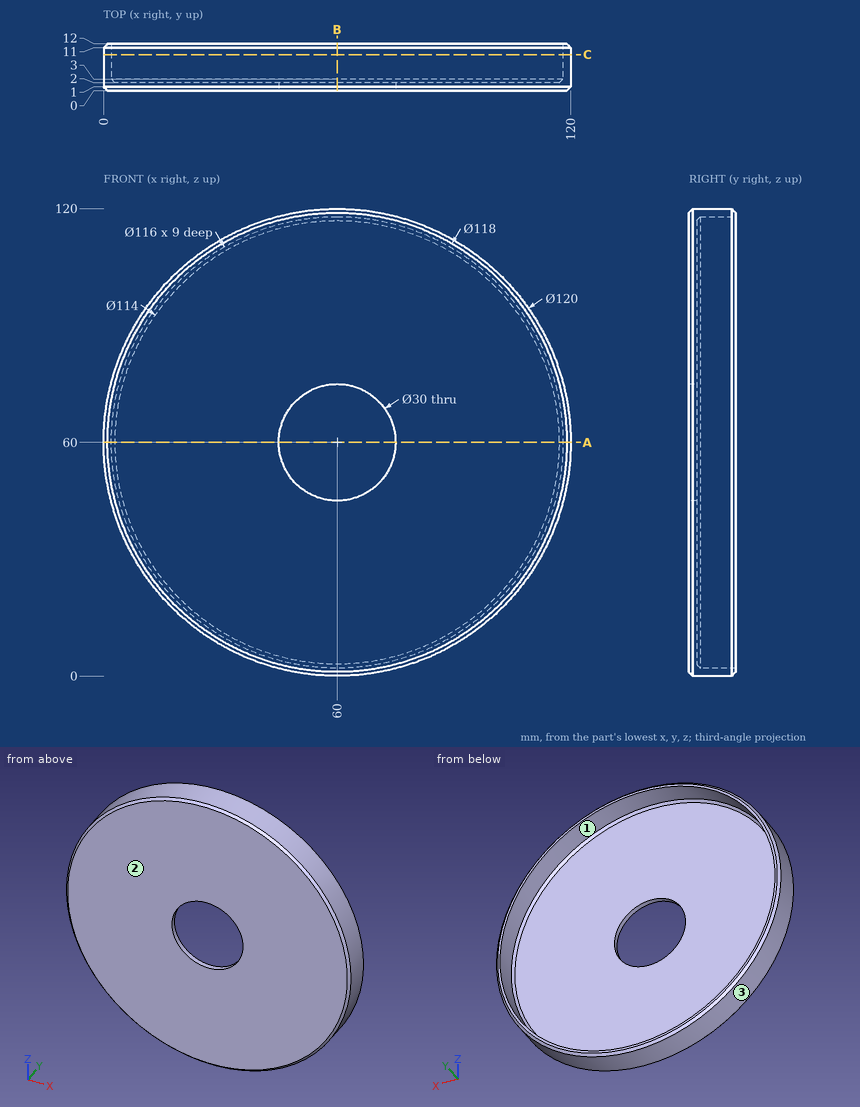
Check sheet for the drawn part. Datum: minimum x, y, z corner. Units: mm. Round coordinates to 2 decimals unless told otherwise and drop trailing zeros. Order: outer loops, then holes, each group sorted by start corner. A loop starts at its lowest first (then second) coordinate and runs counter-clockwise, first axis right, second up. Notation, with made-up numbers: M -30.75,80.25 L -8.75,80.25 A22 ccw -8.75,107.25 Z; hole C -9,18 d9. An arc over 180 degrees is marked long. Write each question's results on one line, items separated by ' | '. Start each with the question number.
1. Draft check along X on the marked faces 1, 2 and 3. Enter one of: pulls with the +X half, pulls with the -X half, needs draft (parallel to the pull), parting line crosses it, or undercut.
2. Cross-section at A-A on z = 60. Record the boundary of the cut face in (x, y).
3. Cross-section at C-C on y = 9.25. Record the boundary of the cut face in (x, z), plus the area to 3 significant figures.
4. Material ranges on L1, parallel to X at y = 1, z = 60; L2, parallel to X at y = 5.5, z = 60; L3, parallel to Y at x = 89.5, z = 104, recorded low to high. Write a range as from..to.
5. Go/stop test with flat-tipped pins: P1, Ø2, axis at x = 30, z = 12, coming from the +Y side; P2, Ø2, axis at x = 40, z = 46, coming from the -Y side; P3, Ø24, axis at x = 60, z = 60, coming from the +Y side; P4, Ø6, axis at x = 55.5, z = 22, coming from the +Y side. Record where each tip stops, or that it passes through.
6. Cross-section at B-B on x = 60. Record the boundary of the cut face in (y, z), plus the area to 3 significant figures.
Resolved:
1) face 1: undercut | face 2: needs draft | face 3: parting line crosses it
2) outline: M 0,1 L 1,0 L 45,0 L 45,2 L 3,2 L 2,3 L 2,12 L 1,12 L 0,11 Z; M 75,0 L 119,0 L 120,1 L 120,11 L 119,12 L 118,12 L 118,3 L 117,2 L 75,2 Z
3) outline: C 60,60 d120; hole C 60,60 d116 | area: 741 mm2
4) L1: 0..45, 75..120 | L2: 0..2, 118..120 | L3: 0..2
5) P1: y = 2.6 | P2: y = 0 | P3: through | P4: y = 2
6) outline: M 0,1 L 1,0 L 11,0 L 12,1 L 12,2 L 3,2 L 2,3 L 2,45 L 0,45 Z; M 0,75 L 2,75 L 2,117 L 3,118 L 12,118 L 12,119 L 11,120 L 1,120 L 0,119 Z | area: 219 mm2
